Source: CAD feature listing. Evaluate the final solid. Frame: model axes, mm. Face numbers are marked on the shaded views. A direction names the side the tool comes from. Round coordinates to 2 decimals unless told otherwise and drop trailing zeros. Loops run counter-clockwise (first coordinate to the right, second up) from the corner with the lowest first, then second, coordinate; pieces in that order, holes last. Notation, with made-up numbers: (46, -34) - (69, -34) arc R13 ccw to (69, -14) - close; hole circle Ø2 at (67.25, -22.5). An arc over 180 degrees is marked (long way). One line per question, with ' | ' between items. Start each with the question number.
1. Mould query, pull axis X, two halves, no side actions, for the marked faces 1, 2 and 3. Classes: pulls with the +X half, pulls with the -X half, needs draft (parallel to the pull), parting line crosses it, or undercut.
2. Ray query, line 1 (X direction, y = -7.25, z = -1.25); line 2 (X direction, y = -12.75, z = -6.75); line 3 (X direction, y = -6.5, z = -4.25). Return the intervals inside material, ascending.
3. Cut plane A-A (x = 34). Return loops of the section in (y, z) (3 decimals), then the cut area to 3 significant figures.
4. Access query for the marked faces 4 and 5. Directions: +Z, -Z, +X, -X, +Y, -Y. A direction counts if a zero-diameter tool reaches every point of the face in a straight line with its end or side. Return the directions, or none.
5. Pin query (flat end, axial travel): pin 1 (2 mm diameter, centred on x = 69, z = -6.5, fed in from +Y); pin 2 (1.5 mm diameter, centred on x = 29.5, y = -14, fed in from -Z); pin 3 (3 mm diameter, centred on y = -13, z = -6, fed in from -X); pin 4 (3 mm diameter, centred on y = -13, z = -8.5, fed in from -X). Return the tip coordinate at first contact, or that it passes through.
```python
from build123d import *

# Parameters (mm, degrees)
F1_DEPTH = 13.97
F2_R     = 9.525
F3_DEPTH = 9.525
F4_R     = 3.556
F5_DEPTH = 9.526
F6_SIZE  = 1.27
F7_R     = 5.08
F8_R     = 1.27


with BuildPart() as f1:
    # F0 (on Front) → F1 (new body)
    with BuildSketch(Plane.XZ):
        with BuildLine():
            ThreePointArc((3.175, 0), (0, -3.175), (-3.175, 0))
            Line((-3.175, 0), (-9.525, 0))
            ThreePointArc((-9.525, 0), (-6.7351920908, -6.7351920908), (0, -9.525))
            ThreePointArc((0, -9.525), (6.7351920908, -6.7351920908), (9.525, 0))
            Line((9.525, 0), (3.175, 0))
        make_face()
        with BuildLine():
            Line((63.373, 0), (9.525, 0))
            ThreePointArc((9.525, 0), (6.7351920908, -6.7351920908), (0, -9.525))
            Line((0, -9.525), (72.898, -9.525))
            ThreePointArc((72.898, -9.525), (66.1628079092, -6.7351920908), (63.373, 0))
        make_face()
        with BuildLine():
            Line((69.723, 0), (63.373, 0))
            ThreePointArc((63.373, 0), (66.1628079092, -6.7351920908), (72.898, -9.525))
            ThreePointArc((72.898, -9.525), (79.6331920908, -6.7351920908), (82.423, 0))
            Line((82.423, 0), (76.073, 0))
            ThreePointArc((76.073, 0), (72.898, -3.175), (69.723, 0))
        make_face()
    extrude(amount=F1_DEPTH)

    # F2 (on face) → F3 (join, through all)
    with BuildSketch(Plane.XY):
        with Locations((14.605, -9.525)):
            Circle(F2_R)
        with Locations((58.293, -9.525)):
            Circle(F2_R)
    extrude(amount=-F3_DEPTH)

    # F4 (on face) → F5 (cut, through all)
    with BuildSketch(Plane.XY):
        with Locations((14.605, -9.525)):
            Circle(F4_R)
        with Locations((58.293, -9.525)):
            Circle(F4_R)
    extrude(amount=-F5_DEPTH, mode=Mode.SUBTRACT)

    # F6
    f6_edges = [f1.edges().sort_by_distance(p)[0] for p in [
        (0, -13.97, -3.175),
        (72.898, -13.97, -3.175),
    ]]
    chamfer(f6_edges, length=F6_SIZE)

    # F7
    f7_edges = [f1.edges().sort_by_distance(p)[0] for p in [
        (6.180773, -13.97, -4.7625),
        (23.029227, -13.97, -4.7625),
        (66.717227, -13.97, -4.7625),
        (49.868773, -13.97, -4.7625),
    ]]
    fillet(f7_edges, radius=F7_R)

    # F8
    f8_edges = [f1.edges().sort_by_distance(p)[0] for p in [
        (36.449, -13.97, -9.525),
        (36.449, 0, -9.525),
    ]]
    fillet(f8_edges, radius=F8_R)


solid = f1.part
```
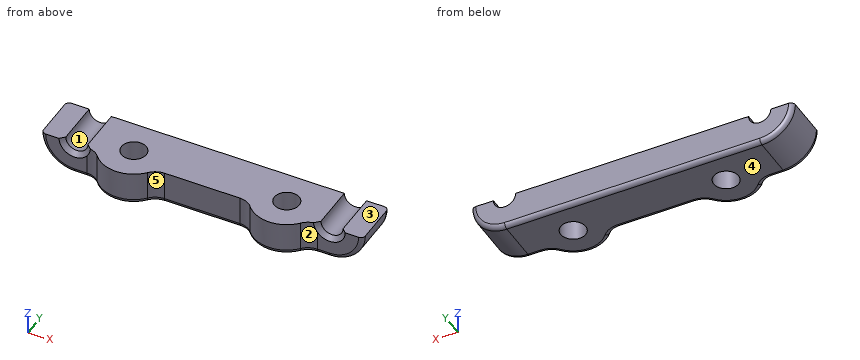
Answers follow:
1) face 1: undercut | face 2: pulls with the +X half | face 3: needs draft
2) line 1: x = -9.44 to -2.92, 2.92 to 11.87, 17.34 to 55.56, 61.03 to 69.98, 75.82 to 82.34 | line 2: x = -6.72 to 13.11, 16.1 to 56.79, 59.79 to 79.62 | line 3: x = -8.52 to 12.74, 16.47 to 56.42, 60.16 to 81.42
3) outline: (-13.97, -8.255) arc R1.27 ccw to (-12.7, -9.525) - (-1.27, -9.525) arc R1.27 ccw to (0, -8.255) - (0, 0) - (-13.97, 0) - close | area: 132 mm2
4) face 4: -Z, +X, -X, +Y, -Y | face 5: +Z, -Z, -Y
5) pin 1: stops at y = 0 | pin 2: stops at z = -9.4 | pin 3: stops at x = -8.38 | pin 4: stops at x = -6.44
